from build123d import *

# Parameters (mm, degrees)
F0_R     = 1.25
F1_DEPTH = 3
F2_R     = 6
F2_R_2   = 4.125
F3_DEPTH = 3
F4_DEPTH = 13.63532


with BuildPart() as f1:
    # F0 (on Top) → F1 (new body)
    with BuildSketch(Plane.XY):
        with BuildLine():
            Line((-20.787705, 6.985428), (-15.100235, 5.07423))
            ThreePointArc((-15.100235, 5.07423), (0, 15.93), (15.100235, 5.07423))
            Line((15.100235, 5.07423), (20.787705, 6.985428))
            ThreePointArc((20.787705, 6.985428), (0, 21.93), (-20.787705, 6.985428))
        make_face()
        with Locations((-16.393861, 9.465)):
            Circle(F0_R, mode=Mode.SUBTRACT)
        with Locations((16.393861, 9.465)):
            Circle(F0_R, mode=Mode.SUBTRACT)
    extrude(amount=F1_DEPTH)

    # F2 (on Top) → F3 (join)
    with BuildSketch(Plane.XY):
        with Locations((6.481612, 20.897385)):
            Circle(F2_R)
        with Locations((6.481612, 20.897385)):
            Circle(F2_R_2, mode=Mode.SUBTRACT)
        with Locations((-6.481612, 20.897385)):
            Circle(F2_R)
        with Locations((-6.481612, 20.897385)):
            Circle(F2_R_2, mode=Mode.SUBTRACT)
    extrude(amount=F3_DEPTH)

    # F2 (on Top) → F4 (cut)
    with BuildSketch(Plane.XY):
        with Locations((-6.481612, 20.897385)):
            Circle(F2_R_2)
        with Locations((6.481612, 20.897385)):
            Circle(F2_R_2)
    extrude(amount=F4_DEPTH, mode=Mode.SUBTRACT)


solid = f1.part
Can you work these out from the model? Positions are in its coordinate system, mm. A direction names the side the tool comes from. Coordinates: 2 decimals unless noted, no trailing zeros. Write each loop counter-clockwise with the first axis right and the second up, starting at its lowest first coordinate (ties: lowest second). Pieces come first, ordered by that corner, then holes. Notation, with made-up numbers: (71.5, 43.25) -> (85.5, 43.25) arc R8 cw to (85.5, 48.25) -> close; hole circle Ø3 at (45, 52.25). An arc over 180 degrees is marked (long way). Write each question's results on one line, items separated by ' | '. Start each with the question number.
Item 1: Please list where these lines run through material, in increasing order: probe 1 along X at (y, z) = (20.75, 0.4); probe 2 along X at (y, z) = (9.75, 2.85); probe 3 along X at (y, z) = (22, 0.9).
Item 2: If we section it at D-D, the plane y = 13.5: Write out the boundary of the cut face in (x, z).
Item 3: If we section it at B-B, the plane y = 18: Write out the boundary of the cut face in (x, z).
Item 4: On a 3-axis mill with a long thin cutter (end or side, diameter ignored), from which of +Z, -Z, +X, -X, +Y, -Y can I reach the whole of each face in a straight line? I mean faces 4 (the cylindrical face through (16.971, 8.356, 1.479)), 5 (the cylindrical face through (-4.713, 15.164, 1.479)), 6 (the cylindrical face through (0.01, 21.93, 1.48)). Say none if no direction works.
Item 5: If we section it at A-A, the plane x = -16: Write out the boundary of the cut face in (y, z), and give its area (3 significant figures).
Item 6: If we section it at C-C, the plane z = 1.7: Write out the boundary of the cut face in (x, y) (3 decimals).
Item 7: I'm going to push flat-ended pins straight in: P1, Ø2, axis at x = 16.39, y = 9.46, coming from the +Z side; P2, Ø1.5, axis at x = 15.5, z = 2, coming from the +Y side; P3, Ø10, axis at x = 6, y = 10.5, coming from the -Z side; P4, Ø1, axis at y = 19.5, z = 1.5, coming from the -X side. Where does each tip first touch, or does it pass through?
Item 8: Thinking about a two-plate mould opening in X: for faces 1 (the cylindrical face through (-7.019, 24.987, 1.479)), 2 (the flat face through (17.904, 6.016, 1.479)), 3 (the flat face through (-17.98, 6.04, 1.48)), which applies, released by +X, released by -X, zero draft, split by the parting line, or undercut?
Answer block:
1) probe 1: -12.48 to -10.6, -2.36 to 2.36, 10.6 to 12.48 | probe 2: -19.64 to -17.61, -15.18 to -12.6, 12.6 to 15.18, 17.61 to 19.64 | probe 3: -12.38 to -10.46, -2.51 to -0.58, 0.58 to 2.51, 10.46 to 12.38
2) outline: (-17.28, 0) -> (-8.46, 0) -> (-8.46, 3) -> (-17.28, 3) -> close; (8.46, 0) -> (17.28, 0) -> (17.28, 3) -> (8.46, 3) -> close
3) outline: (-12.53, 0) -> (-9.42, 0) -> (-9.42, 3) -> (-12.53, 3) -> close; (-3.55, 0) -> (3.55, 0) -> (3.55, 3) -> (-3.55, 3) -> close; (9.42, 0) -> (12.53, 0) -> (12.53, 3) -> (9.42, 3) -> close
4) face 4: +Z, -Z | face 5: +Z, -Z, -Y | face 6: +Z, -Z, +Y
5) outline: (5.38, 0) -> (8.28, 0) -> (8.28, 3) -> (5.38, 3) -> close; (10.65, 0) -> (15, 0) -> (15, 3) -> (10.65, 3) -> close | area: 21.7 mm²
6) outline: (-20.788, 6.985) -> (-15.1, 5.074) arc R15.93 cw to (-5.348, 15.005) arc R6 ccw to (-4.082, 15.398) arc R15.93 cw to (4.082, 15.398) arc R6 ccw to (5.348, 15.005) arc R15.93 cw to (15.1, 5.074) -> (20.788, 6.985) arc R21.93 ccw to (11.936, 18.397) arc R6 ccw (long way) to (0.57, 21.923) arc R21.93 ccw to (-0.57, 21.923) arc R6 ccw (long way) to (-11.936, 18.397) arc R21.93 ccw to start; hole circle Ø2.5 at (-16.394, 9.465); hole circle Ø8.25 at (-6.482, 20.897); hole circle Ø8.25 at (6.482, 20.897); hole circle Ø2.5 at (16.394, 9.465)
7) P1: through | P2: y = 16.23 | P3: z = 0 | P4: x = -12.41
8) face 1: undercut | face 2: released by +X | face 3: released by -X
